Verification items for the finished model (mm, model axes). Give positions to 0.01 mm unless a question says otherwise; leave off trailing zeros. Loops run counter-clockwise (first coordinate to the right, second up) from the corner with the lowest first, then second, coordinate; pieces in that order, holes last. Notation, with made-up numbers: (-3.75, 5.25) - (48.25, 5.25) arc R23 cw to (48.25, 31.25) - close; hole circle Ø11 at (46.25, -8). An arc over 180 degrees is marked (long way). One line per item, written item: value. Start each with the question number.
1. Sectioned sample at A-A (y = -0.75). Record the cut outline in (x, z), plus the area to 3 significant figures.
2. Scan lines: L1, parallel to Y at x = 3.5, z = 96.5; L2, parallel to X at y = 5.25, z = 76; L3, parallel to X at y = 7.25, z = 29. Record each from-to range of solid material in increasing order. Write a range as [from, to].
3. Sectioned sample at B-B (x = 0.25). Record the cut outline in (y, z).
4. Gauge pin test, flat ends, axial feed: pin 1 (1.7 mm diameter, centred on x = -1, z = 42, fed in from -Y); pin 2 (2 mm diameter, centred on x = 0.5, y = -3, fed in from -Z) (3 decimals); pin 3 (6 mm diameter, centred on x = 6, y = -5.5, fed in from +Z); pin 4 (2 mm diameter, centred on x = -1, y = 5.5, fed in from -Z). Record the tip position at first contact, or that the pin passes through.
from build123d import *

# Parameters (mm, degrees)
BOSS_EXTRUDE1_DEPTH = 120
CUT_EXTRUDE1_DEPTH  = 123.065088938
CUT_EXTRUDE2_DEPTH  = 123.065088938


with BuildPart() as part:
    # Sketch1 → Boss-Extrude1 (new body)
    with BuildSketch(Plane.XY):
        Polygon((-2.834320347, 3.893970342), (2.834320347, 3.893970342), (5.5, 6.558849663), (5.5, 8.349069506), (3.1, 8.349069506), (4.75, 9.998574117), (10, 9.998574117), (10, 4.746997406), (8.35, 3.097492795), (8.350720674, 5.497492687), (6.560500912, 5.498030255), (3.894821259, 2.833150935), (3.894821259, -2.833150935), (6.560500912, -5.498030255), (8.350720674, -5.497492687), (8.35, -3.097492795), (10, -4.746997406), (10, -9.998574117), (4.75, -9.998574117), (3.1, -8.349069506), (5.5, -8.349069506), (5.5, -6.558849663), (2.834320347, -3.893970342), (-2.834320347, -3.893970342), (-5.5, -6.558849663), (-5.5, -8.349069506), (-3.1, -8.349069506), (-4.75, -9.998574117), (-10, -9.998574117), (-10, -4.746997406), (-8.35, -3.097492795), (-8.350720674, -5.497492687), (-6.560500912, -5.498030255), (-3.894821259, -2.833150935), (-3.894821259, 2.833150935), (-6.560500912, 5.498030255), (-8.350720674, 5.497492687), (-8.35, 3.097492795), (-10, 4.746997406), (-10, 9.998574117), (-4.75, 9.998574117), (-3.1, 8.349069506), (-5.5, 8.349069506), (-5.5, 6.558849663), align=None)
    extrude(amount=BOSS_EXTRUDE1_DEPTH)

    # Sketch2 → Cut-Extrude1 (cut, through all)
    with BuildSketch(Plane(origin=(0, 9.998574117, 0), x_dir=(1, 0, 0), z_dir=(0, 1, 0))):
        Polygon((-10, -120), (10, -111.715728753), (10, -120), align=None)
    extrude(amount=-CUT_EXTRUDE1_DEPTH, mode=Mode.SUBTRACT)

    # Sketch3 → Cut-Extrude2 (cut, through all)
    with BuildSketch(Plane(origin=(0, 9.998574117, 0), x_dir=(1, 0, 0), z_dir=(0, 1, 0))):
        Polygon((-10, 0), (10, -8.284271247), (10, 0), align=None)
    extrude(amount=-CUT_EXTRUDE2_DEPTH, mode=Mode.SUBTRACT)


solid = part.part
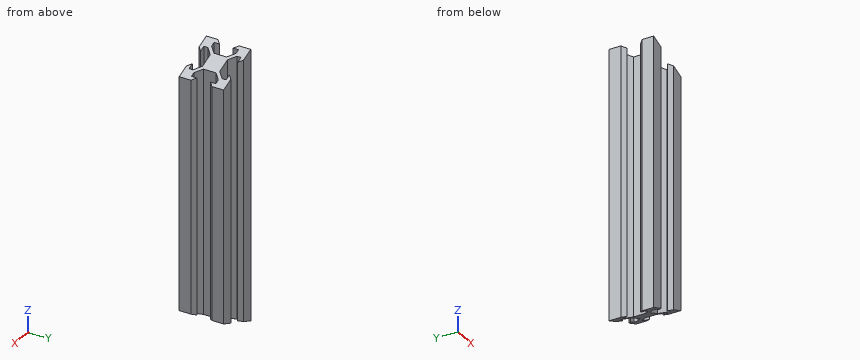
Results are:
1. outline: (-3.89, 2.53) - (3.89, 5.76) - (3.89, 114.24) - (-3.89, 117.47) - close
1. area: 870 mm^2
2. L1: y = [-8.75, -8.35], [-4.56, 4.56], [8.35, 8.75]
2. L2: x = [-10, -8.35], [-6.31, -4.19], [4.19, 6.31], [8.35, 10]
2. L3: x = [-10, -5.5], [5.5, 10]
3. outline: (-3.89, 4.25) - (3.89, 4.25) - (3.89, 115.75) - (-3.89, 115.75) - close
4. pin 1: stops at y = -3.89
4. pin 2: stops at z = 3.935
4. pin 3: stops at z = 114.51
4. pin 4: passes through
